from build123d import *

# Parameters (mm, degrees)
F0_W      = 63.5
F0_H      = 63.5
F1_DEPTH  = 692.15
F2_R      = 4.7625
F3_DEPTH  = 50.8
F5_R      = 6.35
F6_DEPTH  = 60.325
F7_R      = 1.5875
F8_R      = 4.7625
F9_DEPTH  = 50.8
F10_R     = 4.7625
F11_DEPTH = 7.9375


with BuildPart() as f1:
    # F0 (on Top) → F1 (new body)
    with BuildSketch(Plane.XY):
        Rectangle(F0_W, F0_H)
    extrude(amount=-F1_DEPTH)

    # F2 (on face) → F3 (cut)
    with BuildSketch(Plane.XY):
        with Locations((-3.577416998, 3.577416998)):
            Circle(F2_R)
        with Locations((19.05, -19.05)):
            Circle(F2_R)
    extrude(amount=-F3_DEPTH, mode=Mode.SUBTRACT)

    # F5 (on face) → F6 (cut)
    with BuildSketch(Plane(origin=(31.75, -31.75, 0), x_dir=(0.7071067812, 0.7071067812, 0), z_dir=(0.7071067812, -0.7071067812, 0))):
        with Locations((0, -31.75)):
            Circle(F5_R)
    extrude(amount=-F6_DEPTH, mode=Mode.SUBTRACT)

    # F7
    f7_edges = [f1.edges().sort_by_distance(p)[0] for p in [
        (-31.75, -31.75, -346.075),
        (-31.75, 31.75, -346.075),
        (31.75, -31.75, -12.7),
        (31.75, -31.75, -365.125),
        (31.75, 31.75, -346.075),
    ]]
    fillet(f7_edges, radius=F7_R)

    # F8 (on face) → F9 (cut)
    with BuildSketch(Plane(origin=(0, 0, -692.15), x_dir=(1, 0, 0), z_dir=(0, 0, -1))):
        Circle(F8_R)
    extrude(amount=-F9_DEPTH, mode=Mode.SUBTRACT)

    # F10 (on face) → F11 (cut)
    with BuildSketch(Plane.XY):
        with BuildLine():
            Line((31.75, -7.9375), (8.5502364646, 15.0226181746))
            ThreePointArc((8.5502364646, 15.0226181746), (-14.9615861589, 14.9615861589), (-15.0226181746, -8.5502364646))
            Line((-15.0226181746, -8.5502364646), (7.9375, -31.75))
            Line((7.9375, -31.75), (30.1625, -31.75))
            ThreePointArc((30.1625, -31.75), (31.2850320151, -31.2850320151), (31.75, -30.1625))
            Line((31.75, -30.1625), (31.75, -7.9375))
        make_face()
        with Locations((19.05, -19.05)):
            Circle(F10_R, mode=Mode.SUBTRACT)
        with Locations((-3.577416998, 3.577416998)):
            Circle(F10_R, mode=Mode.SUBTRACT)
    extrude(amount=-F11_DEPTH, mode=Mode.SUBTRACT)


solid = f1.part
The listing builds one solid part. Answer for the finished solid, in the listing's coordinates (mm). A direction names the side the tool comes from. Coordinates: 2 decimals unless noted, no trailing zeros. Put each result on its own line as item: value. Start each with the question number.
1. Flat-ended cylindrical pins translate along their axes: P1, Ø10.5, axis at x = -2, y = 3, coming from the +Z side; P2, Ø8.5, axis at x = -3.58, y = 3.58, coming from the +Z side; P3, Ø3, axis at x = 1, y = 0, coming from the -Z side. Find the tip coordinate at first contact, or state that the pin passes through.
2. For a pull along Z with two mould halves and no side action, classify faces 4 (the flat face through (0, 31.75, -341)), 5 (the cylindrical face through (12.56, -8.41, -37.38)), 6 (the flat face through (-22, 8, 0)) as pulls with the +Z half, pulls with the -Z half, needs draft (parallel to the pull), parting line crosses it, or undercut.
3. Consider line 1 (X direction, y = 0, z = -672); line 2 (Y direction, x = -3, z = -44.5). Determine where each line is inside the solid, lowest interval first. Write a range as from..to.
4. Which of the six approach directions +Z, -Z, +X, -X, +Y, -Y give full straight-line access (tool end or side, diameter ignored) to faces 1 (the flat face through (6, -6, -7.938)), 2 (the flat face through (-3.7, -19.99, -3.91)), 3 (the flat face through (20.313, 3.382, -3.913))?
Resolved:
1. P1: stops at z = -7.94
1. P2: stops at z = -50.8
1. P3: stops at z = -641.35
2. face 4: needs draft
2. face 5: undercut
2. face 6: pulls with the +Z half
3. line 1: x = -31.75..-4.76, 4.76..31.75
3. line 2: y = -31.75..-1.15, 8.3..31.75
4. face 1: +Z
4. face 2: +Z, +X
4. face 3: +Z, -Y
